from build123d import *

# Parameters (mm, degrees)
EXTRUDE_1_DEPTH     = 20
FILLET_1_R          = 10
SKETCH_2_R          = 1.5
SKETCH_2_R_2        = 4
CUT_EXTRUDE_1_DEPTH = 71.03570518
SKETCH_3_R          = 3
SKETCH_3_R_2        = 1.5
CUT_EXTRUDE_2_DEPTH = 71.03570518


with BuildPart() as part:
    # 草图1 → 拉伸-薄壁1 (new body)
    with BuildSketch(Plane.XY):
        Polygon((0, 37), (0, 0), (56, 0), (56, 37), (54, 37), (54, 2), (2, 2), (2, 37), align=None)
    extrude(amount=EXTRUDE_1_DEPTH)

    # 圆角1
    fillet_1_edges = [part.edges().sort_by_distance(p)[0] for p in [
        (55, 37, 20),
        (55, 37, 0),
        (1, 37, 0),
        (1, 37, 20),
    ]]
    fillet(fillet_1_edges, radius=FILLET_1_R - 0.0001)  # a hair under: the kernel refuses the full size

    # 草图2 → 切除-拉伸1 (cut, through all)
    with BuildSketch(Plane.ZY):
        with Locations((10, 34)):
            Circle(SKETCH_2_R)
        with Locations((17, 27)):
            Circle(SKETCH_2_R)
        with Locations((10, 20)):
            Circle(SKETCH_2_R)
        with Locations((3, 27)):
            Circle(SKETCH_2_R)
        with Locations((10, 27)):
            Circle(SKETCH_2_R_2)
    extrude(amount=-CUT_EXTRUDE_1_DEPTH, mode=Mode.SUBTRACT)

    # 草图3 → 切除-拉伸2 (cut, through all)
    with BuildSketch(Plane.XZ):
        with Locations(Location((28, 10, 0), (0, 0, 270))):
            Circle(SKETCH_3_R)
        with Locations(Location((32.9495, 14.9495, 0), (0, 0, 270))):
            Circle(SKETCH_3_R_2)
        with Locations(Location((23.0505, 14.9495, 0), (0, 0, 270))):
            Circle(SKETCH_3_R_2)
        with Locations(Location((23.0505, 5.0505, 0), (0, 0, 270))):
            Circle(SKETCH_3_R_2)
        with Locations(Location((32.9495, 5.0505, 0), (0, 0, 270))):
            Circle(SKETCH_3_R_2)
        with Locations(Location((42.8485, 14.9495, 0), (0, 0, 270))):
            Circle(SKETCH_3_R_2)
        with Locations(Location((42.8485, 5.0505, 0), (0, 0, 270))):
            Circle(SKETCH_3_R_2)
        with Locations(Location((13.1515, 5.0505, 0), (0, 0, 270))):
            Circle(SKETCH_3_R_2)
        with Locations(Location((13.1515, 14.9495, 0), (0, 0, 270))):
            Circle(SKETCH_3_R_2)
    extrude(amount=-CUT_EXTRUDE_2_DEPTH, mode=Mode.SUBTRACT)


solid = part.part
The listing builds one solid part. Answer for the finished solid, in the listing's coordinates (mm). A direction names the side the tool comes from. Round coordinates to 2 decimals unless told otherwise and drop trailing zeros. Write each loop counter-clockwise with the first axis right and the second up, starting at its lowest first coordinate (ties: lowest second). Pieces come first, ordered by that corner, then holes. Notation, with made-up numbers: (-34.5, 19) - (-9.5, 19) arc R15 ccw to (-9.5, 34) - close; hole circle Ø9 at (67.25, 58). An arc over 180 degrees is marked (long way). Use a Markdown table: item, result. Add a question column.
1. The part is cut by section D-D (z = 7.75). Write down the section's boundary in (x, y), and give its area (3 significant figures).
2. A flat-ended cylindrical pin translates along its axis: P1, Ø5, axis at x = 13.15, z = 14.95, coming from the -Y side. Find the tip coordinate at first contact, or state that the pin passes through.
3. The part is cut by section C-C (z = 2.25). Write down the section's boundary in (x, y).
4. The part is cut by section A-A (y = 20). Write down the section's boundary in (x, z), and give its area (3 significant figures).
5. A tool of negligible diameter and unlimited length cuts with its end or side. For faces 5 (the face through (54, 16, 10)), 6 (the face through (24.315, 0.986, 14.143)), from which of +Z, -Z, +X, -X, +Y, -Y can it reach the whole face along a straight path? Write none if from no direction.
6. Consider line 1 (Y direction, x = 55.4, z = 10); line 2 (X direction, y = 25, z = 4.25); line 3 (Y direction, x = 3, z = 5.5). Determine where each line is inside the solid, lowest interval first.
7. For a pull along Y with two mould halves and no side action, classify faces 1 (the face through (28, 2, 5)), 2 (the face through (27.9, 1.6, 0)), 3 (the face through (0.99, 29.7, 7.05)), 4 (the face through (0.986, 28.487, 2.805)) as +Y half, -Y half, draft (parallel to the pull), parting line (faces both ways), or undercut.
8. The part is cut by section B-B (y = 7). Write down the section's boundary in (x, z).
Reported:
| question | item | result |
|---|---|---|
| 1 | outline | (0, 0) - (26.02, 0) - (26.02, 2) - (2, 2) - (2, 23.69) - (0, 23.69) - close; (0, 30.31) - (2, 30.31) - (2, 36.74) - (0, 36.74) - close; (29.98, 0) - (56, 0) - (56, 23.69) - (54, 23.69) - (54, 2) - (29.98, 2) - close; (54, 30.31) - (56, 30.31) - (56, 36.74) - (54, 36.74) - close |
| 1 | area | 217 mm^2 |
| 2 | P1 | y = 0 |
| 3 | outline | (0, 0) - (56, 0) - (56, 25.7) - (54, 25.7) - (54, 2) - (2, 2) - (2, 25.7) - (0, 25.7) - close; (0, 28.3) - (2, 28.3) - (2, 33.32) - (0, 33.32) - close; (54, 28.3) - (56, 28.3) - (56, 33.32) - (54, 33.32) - close |
| 4 | outline | (0, 0) - (2, 0) - (2, 8.5) - (0, 8.5) - close; (0, 11.5) - (2, 11.5) - (2, 20) - (0, 20) - close; (54, 0) - (56, 0) - (56, 8.5) - (54, 8.5) - close; (54, 11.5) - (56, 11.5) - (56, 20) - (54, 20) - close |
| 4 | area | 68.0 mm^2 |
| 5 | face 5 | +Z, -Z, +Y |
| 5 | face 6 | +Y, -Y |
| 6 | line 1 | 0 to 18.5, 21.5 to 23, 31 to 32.5, 35.5 to 37 |
| 6 | line 2 | 0 to 2, 54 to 56 |
| 6 | line 3 | 0 to 2 |
| 7 | face 1 | +Y half |
| 7 | face 2 | draft |
| 7 | face 3 | undercut |
| 7 | face 4 | undercut |
| 8 | outline | (0, 0) - (2, 0) - (2, 20) - (0, 20) - close; (54, 0) - (56, 0) - (56, 20) - (54, 20) - close |
